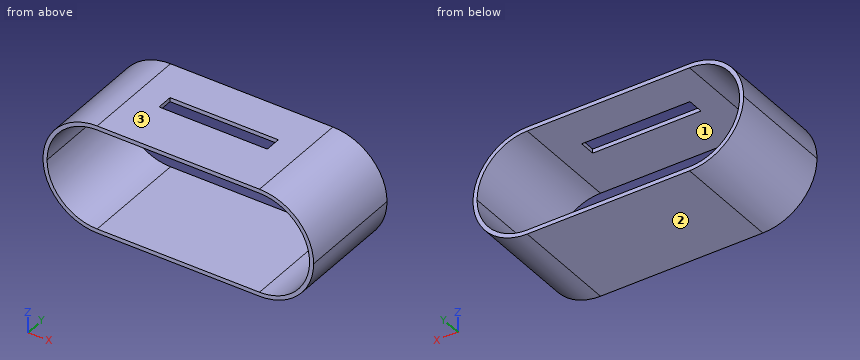
from build123d import *

# Parameters (mm, degrees)
F1_DEPTH = 80
F2_W     = 80
F2_H     = 12
F3_DEPTH = 25


with BuildPart() as f1:
    # F0 (on Front) → F1 (new body)
    with BuildSketch(Plane.XZ):
        with BuildLine():
            Line((60, 40), (-60, 40))
            ThreePointArc((-60, 40), (-88.284271, 28.284271), (-100, 0))
            ThreePointArc((-100, 0), (-88.284271, -28.284271), (-60, -40))
            Line((-60, -40), (60, -40))
            ThreePointArc((60, -40), (88.284271, -28.284271), (100, 0))
            ThreePointArc((100, 0), (88.284271, 28.284271), (60, 40))
        make_face()
        with BuildLine():
            ThreePointArc((-97, 0), (-86.162951, 26.162951), (-60, 37))
            Line((-60, 37), (60, 37))
            ThreePointArc((60, 37), (86.162951, 26.162951), (97, 0))
            ThreePointArc((97, 0), (86.162951, -26.162951), (60, -37))
            Line((60, -37), (-60, -37))
            ThreePointArc((-60, -37), (-86.162951, -26.162951), (-97, 0))
        make_face(mode=Mode.SUBTRACT)
    extrude(amount=F1_DEPTH)

    # F2 (on face) → F3 (cut)
    with BuildSketch(Plane.XY.offset(40)):
        with Locations((0, -36)):
            Rectangle(F2_W, F2_H)
    extrude(amount=-F3_DEPTH, mode=Mode.SUBTRACT)


solid = f1.part
Verification items for the finished model (mm, model axes). Face numbers are marked on the shaded views. Give positions to 0.01 mm unless a question says otherwise; leave off trailing zeros. Loops run counter-clockwise (first coordinate to the right, second up) from the corner with the lowest first, then second, coordinate; pieces in that order, holes last.
1. Cross-section at C-C on y = -19. Record the cut outline in (x, z).
Derived:
outline: (-100, 0) arc R40 ccw to (-60, -40) - (60, -40) arc R40 ccw to (100, 0) arc R40 ccw to (60, 40) - (-60, 40) arc R40 ccw to start; hole (-60, -37) - (60, -37) arc R37 ccw to (60, 37) - (-60, 37) arc R37 ccw to start
2. Material ranges on probe 1 along Z at (x, y) = (-14, -53); probe 2 along X at (y, z) = (-31.5, -0.5); probe 3 along X at (y, z) = (-9.5, 12), recorded low to high.
Derived:
probe 1: z = -40 to -37, 37 to 40
probe 2: x = -100 to -97, 97 to 100
probe 3: x = -98.16 to -95, 95 to 98.16
3. Cross-section at B-B on z = 11. Record the cut outline in (x, y).
Derived:
outline: (-98.46, -80) - (-95.33, -80) - (-95.33, 0) - (-98.46, 0) - close; (95.33, -80) - (98.46, -80) - (98.46, 0) - (95.33, 0) - close
4. Cross-section at D-D on x = -8. Record the cut outline in (y, z).
Derived:
outline: (-80, -40) - (0, -40) - (0, -37) - (-80, -37) - close; (-80, 37) - (-42, 37) - (-42, 40) - (-80, 40) - close; (-30, 37) - (0, 37) - (0, 40) - (-30, 40) - close
5. Cross-section at A-A on x = 65.5. Record the cut outline in (y, z).
Derived:
outline: (-80, -39.62) - (0, -39.62) - (0, -36.59) - (-80, -36.59) - close; (-80, 36.59) - (0, 36.59) - (0, 39.62) - (-80, 39.62) - close
6. Go/stop test with flat-tipped pins: P1, Ø3.5, axis at y = -35.5, z = 38, coming from the +X side; P2, Ø6, axis at y = -50.5, z = -6, coming from the +X side; P3, Ø12, axis at x = -15, z = 27.5, coming from the +Y side; P4, Ø4, axis at y = -47.5, z = 26, coming from the +X side. Record where each tip stops, or that it passes through.
Derived:
P1: stops at x = 76.91
P2: stops at x = 99.89
P3: passes through
P4: stops at x = 92
7. Release check for a two-part mould opening along Z. For the marked faces 1, 2 and 3 record: +Z half, -Z half, draft (parallel to the pull), parting line (faces both ways), or undercut.
Derived:
face 1: undercut
face 2: -Z half
face 3: +Z half
